Part model, mm, in its own coordinate system. A direction names the side the tool comes from. Give positions to 0.01 mm unless a question says otherwise; leave off trailing zeros. Order: outer loops, then holes, each group sorted by start corner. A loop starts at its lowest first (then second) coordinate and runs counter-clockwise, first axis right, second up. Notation, with made-up numbers: M -13.75,26 L 20.25,26 A36 ccw 20.25,64 Z; hole C 41.5,-2 d11. An arc over 180 degrees is marked long. Return JSON: item names as keys, results as strings.
from build123d import *

# Parameters (mm, degrees)
SKETCH2_R          = 3.175
CUT_EXTRUDE1_DEPTH = 57.668552776
CHAMFER1_SIZE      = 1.016


with BuildPart() as part:
    # Sketch1 → Revolve1 (revolve)
    with BuildSketch(Plane.XY, mode=Mode.PRIVATE) as revolve1_sk:
        Polygon((0, 12.7), (31.75, 12.7), (53.747045256, 0), (33.3375, 0), (25.4, 7.9375), (0, 7.9375), align=None)
    revolve(revolve1_sk.sketch.rotate(Axis((0, 0, 0), (1, 0, 0)), 90), axis=Axis((0, 0, 0), (1, 0, 0)))

    # Sketch2 → Cut-Extrude1 (cut, through all)
    with BuildSketch(Plane.XY):
        with Locations(Location((8.89, 0, 0), (0, 0, 180))):
            Circle(SKETCH2_R)
    extrude(amount=CUT_EXTRUDE1_DEPTH, mode=Mode.SUBTRACT)

    # Chamfer1
    chamfer1_edges = [part.edges().sort_by_distance(p)[0] for p in [
        (0, 0, -12.7),
        (0, 0, -7.9375),
    ]]
    chamfer(chamfer1_edges, length=CHAMFER1_SIZE)


solid = part.part
Q1. Band-saw the part on A-A (x = 22.5). Give the cut face in (y, z) (1 decimal), then the cut area to 3 significant figures.
Established:
{"outline": "C 0,0 d25.4; hole C 0,0 d15.9", "area": "309 mm²"}
Q2. Two-plate mould, pull along X, no slides. Class faces 1 (the conical face through (45.347, -1.457, 4.626)), 2 (the flat face through (0, 9, 3)), 3 (the cylindrical face through (5.86, -0.95, 9.95)): +X half, -X half, draft (parallel to the pull), parting line (faces both ways), or undercut.
Established:
{"face 1": "+X half", "face 2": "-X half", "face 3": "undercut"}
Q3. Probe line 1 along Y through (x, z) = (7.5, 0); line 2 along Y through (x, z) = (8.89, 10.6) (3 decimals); line 3 along Z through (x, y) = (15, -6). List the from-to ranges inside material, lowest first.
Established:
{"line 1": "y = -12.7 to -7.94, 7.94 to 12.7", "line 2": "y = -6.995 to -3.175, 3.175 to 6.995", "line 3": "z = -11.19 to -5.2, 5.2 to 11.19"}
Q4. Pin check, flat tips, straight feed: pin 1 (10 mm diameter, centred on x = 44.5, y = 5.5, fed in from +Z); pin 2 (8 mm diameter, centred on y = 1.5, z = -8, fed in from -X); pin 3 (1 mm diameter, centred on x = 48, z = -3, fed in from -Y); pin 4 (2 mm diameter, centred on y = -8, z = -2, fed in from +X). Stop position of each tip, or through.
Established:
{"pin 1": "stops at z = 7.25", "pin 2": "stops at x = 0", "pin 3": "stops at y = -2.33", "pin 4": "stops at x = 41.2"}
Q5. Band-saw the part on D-D (x = 49). Give the cut face in (y, z), then the cut area to 3 significant figures.
Established:
{"outline": "C 0,0 d5.48", "area": "23.6 mm²"}
Q6. Band-saw the part on B-B (x = 42). Give the cut face in (y, z), then the cut area to 3 significant figures.
Established:
{"outline": "C 0,0 d13.56", "area": "145 mm²"}
Q7. 3-axis set-ups, long thin cutter, end or side, ignore diameter. For faces 4 (the cylindrical face through (13.04, 4.83, -6.3)), 5 (the cylindrical face through (16.6, 7.7, -10.1)): which of +Z, -Z, +X, -X, +Y, -Y reach the whole face in a straight line?
Established:
{"face 4": "-X", "face 5": "+X, -X"}
Q8. Band-saw the part on C-C (x = 8.89). Give the cut face in (y, z) (1 decimal).
Established:
{"outline": "M -3.2,7.3 L -3.2,12.3 A12.7 ccw long 3.2,12.3 L 3.2,7.3 A7.9 cw long Z"}
